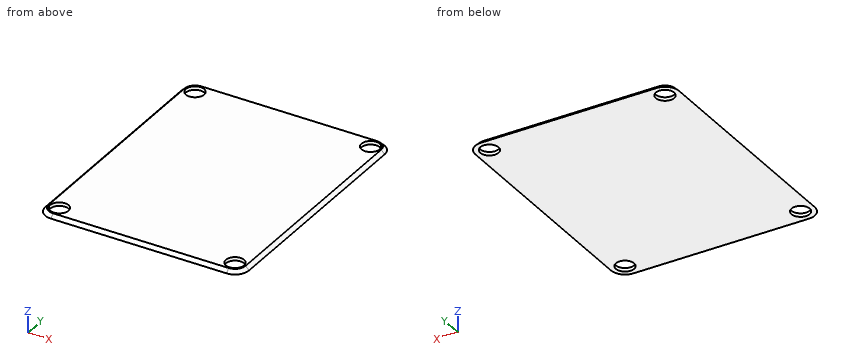
```python
from build123d import *

# Parameters (mm, degrees)
SKETCH034_W      = 60
SKETCH034_H      = 74
SKETCH034_R      = 2.6
EXTRUDE039_DEPTH = 1


with BuildPart() as bevel003:
    # Sweep002: sweep along a path in Sketch041
    with BuildLine(Plane(origin=(0, 0, -2), x_dir=(1, 0, 0), z_dir=(0, 0, -1))) as sweep002_path:
        Line((-25, 35), (25, 35))
        ThreePointArc((25, 35), (27.12132, 34.12132), (28, 32))
        Line((28, 32), (28, -32))
        ThreePointArc((28, -32), (27.12132, -34.12132), (25, -35))
        Line((25, -35), (-25, -35))
        ThreePointArc((-25, -35), (-27.12132, -34.12132), (-28, -32))
        Line((-28, -32), (-28, 32))
        ThreePointArc((-28, 32), (-27.12132, 34.12132), (-25, 35))
    # Sketch040 → Sweep002 (sweep)
    with BuildSketch(Plane.XZ):
        Polygon((-28, 11), (-30, 9), (-30, 1), (-28, -1), (-28, -2), (-33, -2), (-33, 12), (-28, 12), align=None)
    sweep(path=sweep002_path.line)


with BuildPart() as cut:
    # Sketch034 → Extrude039 (new body)
    with BuildSketch(Plane.XY.offset(10)):
        Rectangle(SKETCH034_W, SKETCH034_H)
        with Locations((-25, 32)):
            Circle(SKETCH034_R, mode=Mode.SUBTRACT)
        with Locations((25, 32)):
            Circle(SKETCH034_R, mode=Mode.SUBTRACT)
        with Locations((-25, -32)):
            Circle(SKETCH034_R, mode=Mode.SUBTRACT)
        with Locations((25, -32)):
            Circle(SKETCH034_R, mode=Mode.SUBTRACT)
    extrude(amount=EXTRUDE039_DEPTH)

    # Cut: cut bevel003
    add(bevel003.part, mode=Mode.SUBTRACT)


solid = cut.part
```
CAD build for the part. Positions are in the model's coordinates, mm. Round coordinates to 2 decimals unless told otherwise and drop trailing zeros. Loops run counter-clockwise (first coordinate to the right, second up) from the corner with the lowest first, then second, coordinate; pieces in that order, holes last. Notation, with made-up numbers: M 28,-30 L 36,-30 A18 cw 36,-11 Z; hole C 77,-3 d4. An arc over 180 degrees is marked long. Use a Markdown table: item, result. Add a question column.
(1) Drill centre lines: line 1 (Y direction, x = 25, z = 10.25); line 2 (Y direction, x = 25, z = 10.55). Where is each one in solid material? Low to high.
(2) Cut at A-A (z = 10.4). Give the cut face in (x, y), and give its area (3 significant figures).
(3) Cut at B-B (y = -14). Give the cut face in (x, z).
Geometry says:
| question | item | result |
|---|---|---|
| 1 | line 1 | y = -35.75 to -34.6, -29.4 to 29.4, 34.6 to 35.75 |
| 1 | line 2 | y = -35.45 to -34.6, -29.4 to 29.4, 34.6 to 35.45 |
| 2 | outline | M -28.6,-32 A3.6 ccw -25,-35.6 L 25,-35.6 A3.6 ccw 28.6,-32 L 28.6,32 A3.6 ccw 25,35.6 L -25,35.6 A3.6 ccw -28.6,32 Z; hole C -25,-32 d5.2; hole C -25,32 d5.2; hole C 25,-32 d5.2; hole C 25,32 d5.2 |
| 2 | area | 3,980 mm² |
| 3 | outline | M -29,10 L 29,10 L 28,11 L -28,11 Z |
